Can you work these out from the model? Positions are in its coordinate system, mm. Coordinates: 2 decimals unless noted, no trailing zeros. Order: outer loops, then holes, each group sorted by start corner. A loop starts at its lowest first (then second) coordinate and runs counter-clockwise, first axis right, second up. Notation, with made-up numbers: (61, 76.5) -> (81, 76.5) arc R10 cw to (81, 95.5) -> close; hole circle Ø9 at (3, -32). An arc over 180 degrees is marked (long way). Return JSON: item names as keys, results as strings. Group by question number.
1) If we section it at C-C, the plane x = 92: Please give me the cut outline in (y, z).
2) If we section it at A-A, the plane z = -13: Please give me the cut outline in (x, y).
3) If I drill on probe 1 along X at (y, z) = (0.6, -14); probe 2 along Z at (x, y) = (-3, 2.7); probe 3 along Z at (x, y) = (4.5, 0.35), over which ranges is the centre line in solid material (lowest first)? Write a range as from..to.
4) If we section it at B-B, the plane y = 1.7: State how many separate pieces and enclosed holes the cut face has, then the cut area to 3 significant figures.
5) For pin 1 (0.9 mm diameter, centred on x = -114.5, y = 2, fed in from +Z); pin 2 (0.9 mm diameter, centred on y = 1.5, z = 3, fed in from +X), each with a flat end and sliding along its axis, tell me the tip position at first contact or that it passes through.
6) If we section it at D-D, the plane z = 47.5: Please give me the cut outline in (x, y), then the cut area to 3 significant figures.
from build123d import *

# Parameters (mm, degrees)
SKETCH1_W           = 8.5
SKETCH1_H           = 13.6
BOSS_EXTRUDE1_DEPTH = 3


with BuildPart() as part:
    # Sketch1 → Boss-Extrude1 (new body)
    with BuildSketch(Plane(origin=(0, 0, 0), x_dir=(1, 0, 0), z_dir=(0, 1, 0))):
        Polygon((-111, 30), (-116, 30), (-116, 10), (-111, 10), (-111, -10), (-116, -10), (-116, -30), (-111, -30), (-111, -50), (-66.6, -50), (-66.6, -54), (-22.2, -54), (-22.2, -50), (22.2, -50), (22.2, -54), (66.6, -54), (66.6, -50), (111, -50), (111, -30), (116, -30), (116, -10), (111, -10), (111, 10), (116, 10), (116, 30), (111, 30), (111, 50), (-111, 50), align=None)
        with Locations((0, 13.2)):
            Rectangle(SKETCH1_W, SKETCH1_H, mode=Mode.SUBTRACT)
        with Locations((-50, 13.2)):
            Rectangle(SKETCH1_W, SKETCH1_H, mode=Mode.SUBTRACT)
        with Locations((50, 13.2)):
            Rectangle(SKETCH1_W, SKETCH1_H, mode=Mode.SUBTRACT)
    extrude(amount=BOSS_EXTRUDE1_DEPTH)


solid = part.part
Result sheet:
{
 "1": {"outline": "(0, -50) -> (3, -50) -> (3, 50) -> (0, 50) -> close"},
 "2": {"outline": "(-116, 0) -> (-54.25, 0) -> (-54.25, 3) -> (-116, 3) -> close; (-45.75, 0) -> (-4.25, 0) -> (-4.25, 3) -> (-45.75, 3) -> close; (4.25, 0) -> (45.75, 0) -> (45.75, 3) -> (4.25, 3) -> close; (54.25, 0) -> (116, 0) -> (116, 3) -> (54.25, 3) -> close"},
 "3": {"probe 1": "x = -116..-54.25, -45.75..-4.25, 4.25..45.75, 54.25..116", "probe 2": "z = -50..-20, -6.4..50", "probe 3": "z = -50..50"},
 "4": {"separate pieces": "1", "enclosed holes": "3", "area": "22,600 mm2"},
 "5": {"pin 1": "stops at z = 30", "pin 2": "stops at x = 111"},
 "6": {"outline": "(-111, 0) -> (111, 0) -> (111, 3) -> (-111, 3) -> close", "area": "666 mm2"}
}
